Geometry check sheet. Reference: the model listing, model coordinates, mm. Face numbers are marked on the shaded views. A direction names the side the tool comes from. Coordinates: 2 decimals unless noted, no trailing zeros. Write each loop counter-clockwise with the first axis right and the second up, starting at its lowest first coordinate (ties: lowest second). Pieces come first, ordered by that corner, then holes. Notation, with made-up numbers: (22, 33.25) -> (42, 33.25) arc R27 ccw to (42, 50.25) -> close; hole circle Ø2 at (-6.75, -28.75). An arc over 180 degrees is marked (long way). Use a Markdown table: item, result.
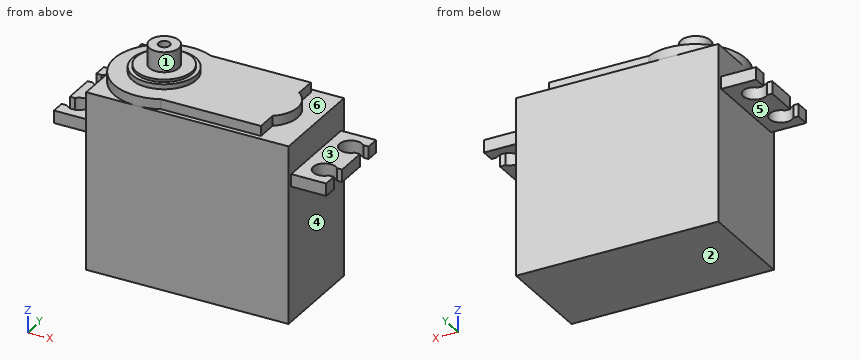
Solid Edge part; units mm, degrees
sketch "Sketch1" plane through (0, 0, 0) normal (0, -1, 0) x (1, 0, 0)
  line L0 (0.6959, 36.2554) -> (0.6959, 0.7554)
  line L1 (0.6959, 0.7554) -> (41.1959, 0.7554)
  line L2 (41.1959, 36.2554) -> (41.1959, 0.7554)
  line L3 (0.6959, 36.2554) -> (41.1959, 36.2554)
  line L4 (-6.3041, 30.2554) -> (0.6959, 30.2554)
  line L5 (0.6959, 30.2554) -> (0.6959, 27.7554)
  line L6 (-6.3041, 27.7554) -> (0.6959, 27.7554)
  line L7 (-6.3041, 27.7554) -> (-6.3041, 30.2554)
  line L8 (48.1959, 27.7554) -> (41.1959, 27.7554)
  line L9 (41.1959, 30.2554) -> (41.1959, 27.7554)
  line L10 (48.1959, 30.2554) -> (41.1959, 30.2554)
  line L11 (48.1959, 27.7554) -> (48.1959, 30.2554)
extrude "Protrusion1" add sketch "Sketch1" against normal blind 20
sketch "Sketch2" plane through (-2.8041, 10, 30.2554) normal (0, 0, 1) x (1, 0, 0)
  line L0 (-3.5, 8.964) -> (3.5, 8.964)
  line L1 (3.5, 8.964) -> (3.5, 10.8897)
  line L2 (3.5, 10.8897) -> (-4.9405, 10.8897)
  line L3 (-4.9405, 10.8897) -> (-4.7039, -10.9349)
  line L4 (-4.7039, -10.9349) -> (3.5, -10.9349)
  line L5 (3.5, -10.9349) -> (3.5, -9.036)
  line L6 (3.5, -9.036) -> (-3.5, -9.036)
  line L7 (-3.5, -9.036) -> (-3.5, -6.286)
  line L8 (-3.5, -6.286) -> (-2.4891, -6.286)
  arc A0 (-2.4891, -6.286) -> (-2.4891, -3.286) centre (-0.812, -4.786) ccw
  line L9 (-2.4891, -3.286) -> (-3.5, -3.286)
  line L10 (-3.5, -3.286) -> (-3.5, 3.1474)
  line L11 (-3.5, 3.1474) -> (-2.4271, 3.1474)
  arc A1 (-2.4271, 3.1474) -> (-2.4271, 6.2806) centre (-0.812, 4.714) ccw
  line L12 (-2.4271, 6.2806) -> (-3.5, 6.2806)
  line L13 (-3.5, 6.2806) -> (-3.5, 8.964)
extrude "Cutout1" cut sketch "Sketch2" against normal up to vertex (2.5 mm away)
mirror "Mirror1" about plane through (20.9459, 10, 18.5054) normal (-1, 0, 0) of "Cutout1"
sketch "Sketch3" plane through (20.9459, 10, 36.2554) normal (0, 0, 1) x (1, 0, 0)
  arc A0 (-5.812, 8.964) -> (-5.812, -9.036) centre (-10.1709, -0.036) ccw
  line L0 (-5.812, -9.036) -> (14.188, -9.036)
  line L1 (14.188, -9.036) -> (14.188, -4.836)
  arc A1 (14.188, -4.836) -> (14.188, 4.764) centre (10.588, -0.036) ccw
  line L2 (14.188, 4.764) -> (14.188, 8.964)
  line L3 (14.188, 8.964) -> (-5.812, 8.964)
extrude "Protrusion2" add sketch "Sketch3" along normal up to vertex (2 mm away)
sketch "Sketch4" plane through (19.1544, 9.964, 38.2554) normal (0, 0, 1) x (1, 0, 0)
  circle A0 centre (-8.3794, 0) radius 6.4
extrude "Protrusion3" add sketch "Sketch4" along normal up to vertex (1 mm away)
sketch "Sketch5" plane through (10.775, 9.964, 39.2554) normal (0, 0, 1) x (1, 0, 0)
  circle A0 centre (0, 0) radius 5.575
extrude "Protrusion4" add sketch "Sketch5" along normal up to vertex (0.5 mm away)
sketch "Sketch6" plane through (10.775, 9.964, 39.7554) normal (0, 0, 1) x (1, 0, 0)
  circle A0 centre (0, 0) radius 2.95
extrude "Protrusion5" add sketch "Sketch6" along normal up to vertex (4 mm away)
sketch "Sketch7" plane through (10.775, 9.964, 43.7554) normal (0, 0, 1) x (1, 0, 0)
  circle A0 centre (0, 0) radius 1.15
extrude "Cutout3" cut sketch "Sketch7" against normal up to vertex (4 mm away)
Item 1: Thickness scan on L1, parallel to Y at x = 34.5, z = 30.5; L2, parallel to X at y = 14.5, z = 27; L3, parallel to Z at x = 30, y = 15.5. Record the ranges inside material, lowest first. Write a range as [from, to].
Answer block:
| item | result |
|---|---|
| L1 | y = [0, 20] |
| L2 | x = [0.7, 41.2] |
| L3 | z = [0.76, 38.26] |
Item 2: Section check A-A on z = 19.5. Record the boundary of the cut face in (x, y), then the cut area to 3 significant figures.
Answer block:
| item | result |
|---|---|
| outline | (0.7, 0) -> (41.2, 0) -> (41.2, 20) -> (0.7, 20) -> close |
| area | 810 mm^2 |
Item 3: Section check C-C on x = -0.5. Record the boundary of the cut face in (y, z).
Answer block:
| item | result |
|---|---|
| outline | (0.96, 27.76) -> (18.96, 27.76) -> (18.96, 30.26) -> (0.96, 30.26) -> close |
Item 4: Section check B-B on y = 2.25. Record the boundary of the cut face in (x, z), then the cut area to 3 significant figures.
Answer block:
| item | result |
|---|---|
| outline | (-6.3, 27.76) -> (0.7, 27.76) -> (0.7, 0.76) -> (41.2, 0.76) -> (41.2, 27.76) -> (48.2, 27.76) -> (48.2, 30.26) -> (41.2, 30.26) -> (41.2, 36.26) -> (35.13, 36.26) -> (35.13, 38.26) -> (4.41, 38.26) -> (4.41, 36.26) -> (0.7, 36.26) -> (0.7, 30.26) -> (-6.3, 30.26) -> close |
| area | 1,530 mm^2 |
Item 5: Mould release check, pull along Z, two halves, no side actions. Record for the marked faces 4, 5 and 6: +Z half, -Z half, draft (parallel to the pull), parting line (faces both ways), or undercut.
Answer block:
| item | result |
|---|---|
| face 4 | draft |
| face 5 | -Z half |
| face 6 | +Z half |
Item 6: Depth check by flat-ended pin: P1, Ø4, axis at x = 29, y = 3.5, coming from the +Z side; P2, Ø0.5, axis at x = 48, z = 29, coming from the -Y side; P3, Ø5.5, axis at x = -3, y = 7, coming from the +Z side. Enter the tip coordinate at first touch or a pass-through.
Answer block:
| item | result |
|---|---|
| P1 | stops at z = 38.26 |
| P2 | stops at y = 0.96 |
| P3 | stops at z = 30.26 |
Item 7: Tool access check on the marked faces 1, 2 and 3. Record the directions out of +Z, -Z, +X, -X, +Y, -Y that give a thin tool (end or side, any length) a straight path to the whole face; none if there is none.
Answer block:
| item | result |
|---|---|
| face 1 | +Z |
| face 2 | -Z, +X, -X, +Y, -Y |
| face 3 | +Z, +X, +Y, -Y |
